Part print with two shaded views. Sizes in mm from the minimum x, y, z corner. A direction names the side the tool comes from. Give positions to 0.01 mm unless a question says otherwise; leave off trailing zeros. Write each loop counter-clockwise with the first axis right and the second up, starting at its lowest first coordinate (ties: lowest second). Pieces come first, ordered by that corner, then holes. Notation, with made-up numbers: (-12.5, 62.5) -> (43.5, 62.5) arc R16 ccw to (43.5, 77.5) -> close; hole circle Ø2 at (-10, -15.75). An arc over 180 degrees is marked (long way). Use one line per item in the form item = value. Start each with the question number.
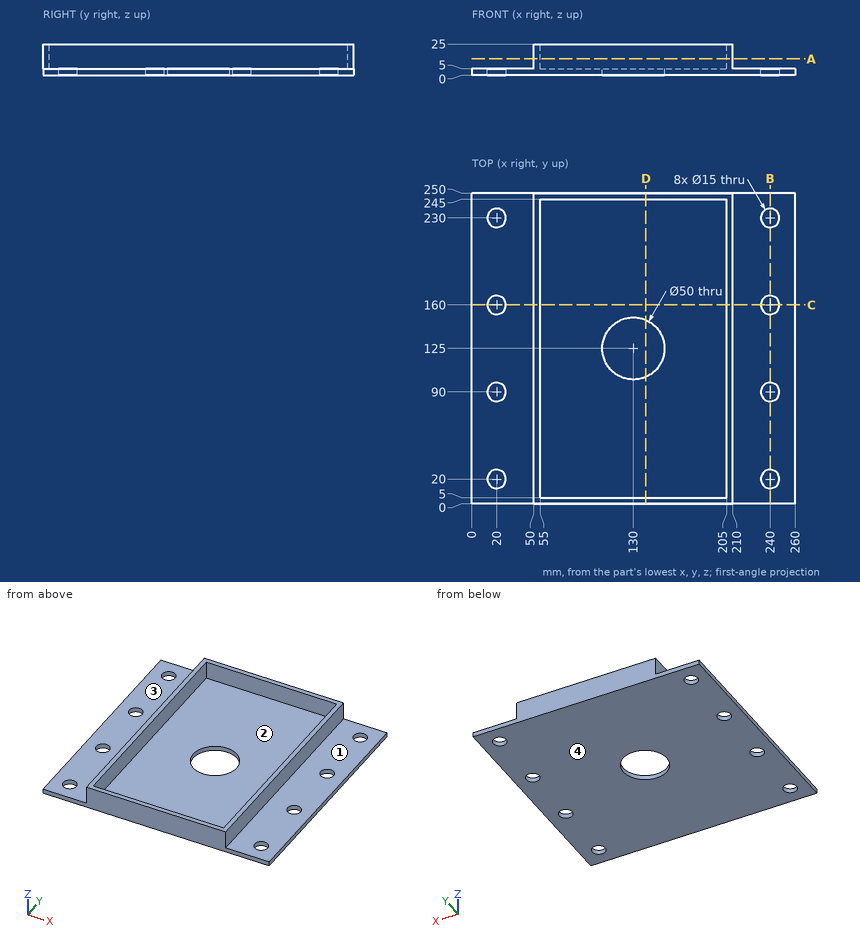
1) Cut at C-C (y = 160). Give the cut face in (x, z).
2) Cut at A-A (z = 13). Give the cut face in (x, y), and give its area (3 significant figures).
3) 3-axis set-ups, long thin cutter, end or side, ignore diameter. For the marked faces 3 and 4: which of +Z, -Z, +X, -X, +Y, -Y reach the whole face in a straight line?
4) Cut at B-B (x = 240). Give the cut face in (y, z).
5) Wall check: line 1 along Y through (x, z) = (20, 2.3); line 2 along X through (y, z) = (12, 17); line 3 along Y through (x, z) = (156, 14.5). Give the ranges that are in metal, low to high. Write a range as from..to.
6) Cut at D-D (x = 140). Give the cut face in (y, z).
7) Two-plate mould, pull along X, no slides. Class the marked faces 1 and 2: released by +X, released by -X, zero draft, split by the parting line, or undercut.
8) Pin check, flat tips, straight feed: pin 1 (9 mm diameter, centred on x = 240, y = 20, fed in from -Z); pin 2 (6 mm diameter, centred on y = 83, z = 18.5, fed in from -X); pin 3 (17 mm diameter, centred on x = 240, y = 230, fed in from +Z). Stop position of each tip, or through.
Final values:
q1.outline = (0, 0) -> (12.5, 0) -> (12.5, 5) -> (0, 5) -> close; (27.5, 0) -> (232.5, 0) -> (232.5, 5) -> (210, 5) -> (210, 25) -> (205, 25) -> (205, 5) -> (55, 5) -> (55, 25) -> (50, 25) -> (50, 5) -> (27.5, 5) -> close; (247.5, 0) -> (260, 0) -> (260, 5) -> (247.5, 5) -> close
q2.outline = (50, 0) -> (210, 0) -> (210, 250) -> (50, 250) -> close; hole (55, 5) -> (205, 5) -> (205, 245) -> (55, 245) -> close
q2.area = 4,000 mm^2
q3.face_3 = +Z, -X, +Y, -Y
q3.face_4 = -Z, +X, -X, +Y, -Y
q4.outline = (0, 0) -> (12.5, 0) -> (12.5, 5) -> (0, 5) -> close; (27.5, 0) -> (82.5, 0) -> (82.5, 5) -> (27.5, 5) -> close; (97.5, 0) -> (152.5, 0) -> (152.5, 5) -> (97.5, 5) -> close; (167.5, 0) -> (222.5, 0) -> (222.5, 5) -> (167.5, 5) -> close; (237.5, 0) -> (250, 0) -> (250, 5) -> (237.5, 5) -> close
q5.line_1 = 0..12.5, 27.5..82.5, 97.5..152.5, 167.5..222.5, 237.5..250
q5.line_2 = 50..55, 205..210
q5.line_3 = 0..5, 245..250
q6.outline = (0, 0) -> (102.09, 0) -> (102.09, 5) -> (5, 5) -> (5, 25) -> (0, 25) -> close; (147.91, 0) -> (250, 0) -> (250, 25) -> (245, 25) -> (245, 5) -> (147.91, 5) -> close
q7.face_1 = zero draft
q7.face_2 = undercut
q8.pin_1 = through
q8.pin_2 = 50
q8.pin_3 = 5
